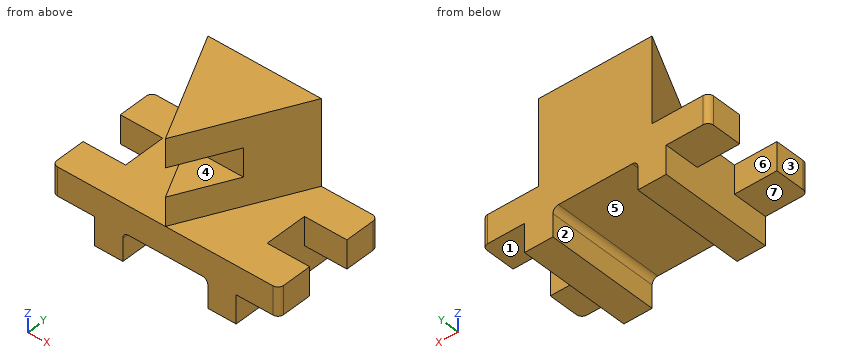
```python
from build123d import *

# Parameters (mm, degrees)
F0_W      = 203.2
F0_H      = 25.4
F1_DEPTH  = 50.8
F2_R      = 5.08
F4_DEPTH  = 76.2
F5_W      = 101.6
F5_H      = 25.4
F6_DEPTH  = 63.5
F7_W      = 50.8
F7_H      = 25.4
F8_DEPTH  = 50.801
F9_W      = 38.1
F9_H      = 25.4
F10_DEPTH = 38.1
F11_W     = 38.1
F11_H     = 25.4
F12_DEPTH = 38.1
F13_W     = 76.2
F13_H     = 25.4
F14_DEPTH = 101.601
F15_R     = 5.08


with BuildPart() as f1:
    # F0 (on Front) → F1 (new body, symmetric)
    with BuildSketch(Plane.XZ):
        with Locations((0, 12.7)):
            Rectangle(F0_W, F0_H)
    extrude(amount=F1_DEPTH, both=True)

    # F2
    f2_edges = [f1.edges().sort_by_distance(p)[0] for p in [
        (101.6, -50.8, 12.7),
        (101.6, 50.8, 12.7),
        (-101.6, -50.8, 12.7),
        (-101.6, 50.8, 12.7),
    ]]
    fillet(f2_edges, radius=F2_R)

    # F3 (on face) → F4 (join)
    with BuildSketch(Plane.XY.offset(25.4)):
        Polygon((50.8, 50.8), (-50.8, 50.8), (0, -50.8), align=None)
    extrude(amount=F4_DEPTH)

    # F5 (on Right) → F6 (join, symmetric)
    with BuildSketch(Plane.YZ):
        with Locations((0, -12.7)):
            Rectangle(F5_W, F5_H)
    extrude(amount=F6_DEPTH, both=True)

    # F7 (on Front) → F8 (cut, through all)
    with BuildSketch(Plane.XZ):
        with Locations((0, 63.5)):
            Rectangle(F7_W, F7_H)
    extrude(amount=F8_DEPTH, mode=Mode.SUBTRACT)

    # F9 (on face) → F10 (cut)
    with BuildSketch(Plane(origin=(-101.6, 0, 0), x_dir=(0, -1, 0), z_dir=(-1, 0, 0))):
        with Locations((0, 12.7)):
            Rectangle(F9_W, F9_H)
    extrude(amount=-F10_DEPTH, mode=Mode.SUBTRACT)

    # F11 (on face) → F12 (cut)
    with BuildSketch(Plane.YZ.offset(101.6)):
        with Locations((0, 12.7)):
            Rectangle(F11_W, F11_H)
    extrude(amount=-F12_DEPTH, mode=Mode.SUBTRACT)

    # F13 (on face) → F14 (cut, through all)
    with BuildSketch(Plane.XZ.offset(50.8)):
        with Locations((0, -12.7)):
            Rectangle(F13_W, F13_H)
    extrude(amount=-F14_DEPTH, mode=Mode.SUBTRACT)

    # F15
    f15_edges = [f1.edges().sort_by_distance(p)[0] for p in [
        (-38.1, 0, 0),
        (38.1, 0, 0),
    ]]
    fillet(f15_edges, radius=F15_R)


solid = f1.part
```
Input: part model. Units: mm. Frame: model coordinates. Face numbers are marked on the shaded views. A direction names the side the tool comes from. Give positions to 0.01 mm unless a question says otherwise; leave off trailing zeros. Order: outer loops, then holes, each group sorted by start corner. A loop starts at its lowest first (then second) coordinate and runs counter-clockwise, first axis right, second up. Notation, with made-up numbers: M 35,-16 L 92,-16 A21 ccw 92,7 Z; hole C 9,68.25 d4. An arc over 180 degrees is marked long. Return JSON: item names as keys, results as strings.
Item 1: Cut plane D-D (x = 30.5). Return loops of the section in (y, z).
Solutions:
{"outline": "M -50.8,0 L 50.8,0 L 50.8,101.6 L 10.2,101.6 L 10.2,25.4 L -50.8,25.4 Z"}
Item 2: Pull-direction query (X, two-part tool) for the marked faces 1, 2 and 3; classes: +X half, -X half, draft (parallel to the pull), parting line (faces both ways), or undercut.
Solutions:
{"face 1": "draft", "face 2": "undercut", "face 3": "-X half"}
Item 3: Cut plane A-A (y = -23). Return loops of the section in (x, z), then the cut area to 3 significant figures.
Solutions:
{"outline": "M -101.6,0 L -63.5,0 L -63.5,-25.4 L -38.1,-25.4 L -38.1,-5.08 A5.08 cw -33.02,0 L 33.02,0 A5.08 cw 38.1,-5.08 L 38.1,-25.4 L 63.5,-25.4 L 63.5,0 L 101.6,0 L 101.6,25.4 L 13.9,25.4 L 13.9,50.8 L -13.9,50.8 L -13.9,25.4 L -101.6,25.4 Z; M -13.9,76.2 L 13.9,76.2 L 13.9,101.6 L -13.9,101.6 Z", "area": "7,870 mm^2"}
Item 4: Ray query, probe 1 along X at (y, z) = (-0.5, -15); probe 2 along Y at (x, z) = (84, 23); probe 3 along Z at (x, y) = (15, -15.5). Return the intervals inside material, ascending.
Solutions:
{"probe 1": "-63.5 to -38.1, 38.1 to 63.5", "probe 2": "-50.8 to -19.05, 19.05 to 50.8", "probe 3": "0 to 50.8, 76.2 to 101.6"}
Item 5: First-contact query: P1, Ø4, axis at y = 17.5, z = -1.5, coming from the -X side; P2, Ø4, axis at y = -33, z = 48.5, coming from the -X side; P3, Ø20, axis at x = 4, y = 23.5, coming from the -Z side. Flat tips, straight axial feed; report the tip coordinate or a pass-through.
Solutions:
{"P1": "x = -63.5", "P2": "x = -9.9", "P3": "z = 0"}
Item 6: Cut plane B-B (x = 67.5). Return loops of the section in (y, z).
Solutions:
{"outline": "M -50.8,0 L -19.05,0 L -19.05,25.4 L -50.8,25.4 Z; M 19.05,0 L 50.8,0 L 50.8,25.4 L 19.05,25.4 Z"}
Item 7: Cut plane C-C (y = 22). Return loops of the section in (x, z).
Solutions:
{"outline": "M -101.6,0 L -63.5,0 L -63.5,-25.4 L -38.1,-25.4 L -38.1,-5.08 A5.08 cw -33.02,0 L 33.02,0 A5.08 cw 38.1,-5.08 L 38.1,-25.4 L 63.5,-25.4 L 63.5,0 L 101.6,0 L 101.6,25.4 L 36.4,25.4 L 36.4,101.6 L -36.4,101.6 L -36.4,25.4 L -101.6,25.4 Z"}
Item 8: Access query for the marked faces 4, 5, 6 and 7. Directions: +Z, -Z, +X, -X, +Y, -Y. A direction counts if a zero-diameter tool reaches every point of the face in a straight line with its end or side. Return the directions, or none.
Solutions:
{"face 4": "+X, -X, -Y", "face 5": "-Z, +Y, -Y", "face 6": "+Z, -Z, -X", "face 7": "-Z, -X, +Y, -Y"}
